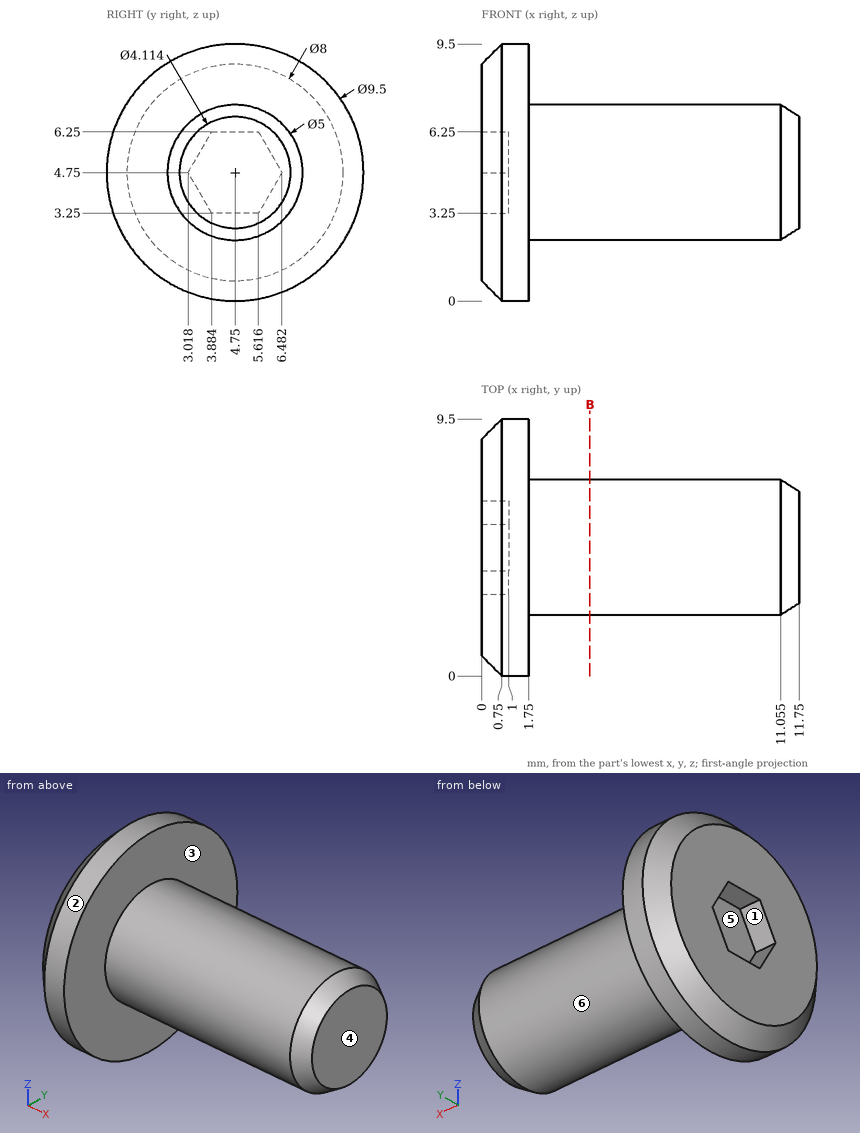
Geometry check sheet. Reference: drawing and pictorial views, mm from the part's lowest x, y, z. A direction names the side the tool comes from. Coordinates: 2 decimals unless noted, no trailing zeros. Loops run counter-clockwise (first coordinate to the right, second up) from the corner with the lowest first, then second, coordinate; pieces in that order, holes last.
1) Material ranges on probe 1 along X at (y, z) = (2.75, 1.5); probe 2 along Z at (x, y) = (9, 6.75); probe 3 along X at (y, z) = (8.75, 3.5), recorded low to high.
2) Release check for a two-part mould opening along Z. For the marked faces 4, 5 and 6 record: released by +Z, released by -Z, zero draft, split by the parting line, or undercut.
3) Gauge pin test, flat ends, axial feed: pin 1 (2 mm diameter, centred on x = 3.5, y = 1, fed in from +Z); pin 2 (5 mm diameter, centred on x = 5.5, y = 4, fed in from +Z); pin 3 (2 mm diameter, centred on x = 9, z = 3, fed in from +Y) (1 decimal); pin 4 (5 mm diameter, centred on x = 3, z = 1, fed in from -Y). Record the tip position at first contact, or that the pin passes through.
4) Sectioned sample at B-B (x = 4). Record the boundary of the cut face in (y, z).
5) Access from +Z, -Z, +X, -X, +Y, -Y to the whole of each face (thin tool, end or side, straight path). Record for the marked faces 1, 2 and 3.
Check sheet entries:
1. probe 1: x = 0 to 1.75
1. probe 2: z = 3.25 to 6.25
1. probe 3: x = 0.19 to 1.75
2. face 4: zero draft
2. face 5: undercut
2. face 6: split by the parting line
3. pin 1: passes through
3. pin 2: stops at z = 7.25
3. pin 3: stops at y = 7.1
3. pin 4: stops at y = 0.27
4. outline: circle Ø5 at (4.75, 4.75)
5. face 1: -X
5. face 2: +X, -X
5. face 3: +X
